Autodesk Inventor part; units mm, degrees
ref_plane "YZ Plane" through (0, 0, 0) normal (1, 0, 0) x (0, 1, 0)
ref_plane "XZ Plane" through (0, 0, 0) normal (0, 1, 0) x (-1, 0, 0)
ref_plane "XY Plane" through (0, 0, 0) normal (0, 0, 1) x (1, 0, 0)
sketch "Esboço1" plane through (0, 0, 0) normal (0, 0, 1) x (1, 0, 0)
  line L0 (0, 0) -> (100, 0)
  line L1 (100, 0) -> (100, -100)
  line L2 (100, -100) -> (0, -100)
  line L3 (0, -100) -> (0, 0)
  dimension "d0" = 100
  dimension "d1" = 100
extrude "Extrusão1" add sketch "Esboço1" along normal blind 3
sketch "Esboço2" plane through (0, 0, 3) normal (0, 0, 1) x (1, 0, 0)
  line L0 (0, 0) -> (0, -100)
  line L1 (0, 0) -> (9.75, 0)
  line L2 (100, 0) -> (0, 0)
  line L3 (9.75, 0) -> (9.75, -10)
  line L4 (9.75, 0) -> (21.25, 0)
  line L5 (21.25, 0) -> (32.75, 0)
  line L6 (32.75, 0) -> (44.25, 0)
  line L7 (44.25, 0) -> (55.75, 0)
  line L8 (55.75, 0) -> (67.25, 0)
  line L9 (67.25, 0) -> (78.75, 0)
  line L10 (78.75, 0) -> (90.25, 0)
  line L11 (90.25, 0) -> (100, 0)
  line L12 (21.25, 0) -> (21.25, -10)
  line L13 (9.75, -10) -> (9.75, -37.6)
  line L14 (9.75, -37.6) -> (21.25, -37.6)
  line L15 (21.25, -37.6) -> (32.75, -37.6)
  line L16 (32.75, -37.6) -> (44.25, -37.6)
  line L17 (44.25, -37.6) -> (55.75, -37.6)
  line L18 (55.75, -37.6) -> (67.25, -37.6)
  line L19 (67.25, -37.6) -> (78.75, -37.6)
  line L20 (78.75, -37.6) -> (90.25, -37.6)
  line L21 (90.25, -37.6) -> (90.25, -10)
  line L22 (90.25, -10) -> (78.75, -10)
  line L23 (78.75, -10) -> (67.25, -10)
  line L24 (67.25, -10) -> (55.75, -10)
  line L25 (55.75, -10) -> (44.25, -10)
  line L26 (44.25, -10) -> (32.75, -10)
  line L27 (32.75, -10) -> (21.25, -10)
  circle A0 centre (9.75, -10) radius 1.5
  circle A1 centre (9.75, -37.6) radius 1.5
  circle A2 centre (32.75, -10) radius 1.5
  circle A3 centre (55.75, -10) radius 1.5
  circle A4 centre (78.75, -10) radius 1.5
  circle A5 centre (78.75, -37.6) radius 1.5
  circle A6 centre (55.75, -37.6) radius 1.5
  circle A7 centre (32.75, -37.6) radius 1.5
  line L28 (21.25, -10) -> (21.25, -20)
  circle A8 centre (21.25, -20) radius 1.5
  line L29 (21.25, -20) -> (21.25, -47.6)
  line L30 (21.25, -47.6) -> (44.25, -47.6)
  line L31 (44.25, -47.6) -> (67.25, -47.6)
  line L32 (67.25, -47.6) -> (90.25, -47.6)
  line L33 (90.25, -47.6) -> (90.25, -20)
  line L34 (90.25, -20) -> (67.25, -20)
  line L35 (67.25, -20) -> (44.25, -20)
  circle A9 centre (21.25, -47.6) radius 1.5
  circle A10 centre (44.25, -47.6) radius 1.5
  circle A11 centre (67.25, -47.6) radius 1.5
  circle A12 centre (90.25, -47.6) radius 1.5
  circle A13 centre (90.25, -20) radius 1.5
  circle A14 centre (67.25, -20) radius 1.5
  circle A15 centre (44.25, -20) radius 1.5
  dimension "d4" = 9.75
  dimension "d5" = 10
  dimension "d7" = 11.5
  dimension "d8" = 11.5
  dimension "d9" = 11.5
  dimension "d10" = 11.5
  dimension "d11" = 11.5
  dimension "d12" = 11.5
  dimension "d13" = 11.5
  dimension "d14" = 27.6
  dimension "d16" = 3
  dimension "d17" = 3
  dimension "d19" = 3
  dimension "d21" = 3
  dimension "d23" = 3
  dimension "d26" = 3
  dimension "d28" = 3
  dimension "d30" = 3
  dimension "d101" = 10
  dimension "d102" = 3
  dimension "d103" = 27.6
  dimension "d104" = 23
  dimension "d105" = 23
  dimension "d106" = 23
  dimension "d107" = 27.6
  dimension "d108" = 23
  dimension "d109" = 23
  dimension "d110" = 3
  dimension "d111" = 3
  dimension "d112" = 3
  dimension "d113" = 3
  dimension "d114" = 3
  dimension "d115" = 3
  dimension "d116" = 3
extrude "Extrusão6" add sketch "Esboço2" along normal blind 15 contours A15 | A14 L35 L34 | L34 L35 A14 | A0 L13 L3 | L3 L13 A0 | A2 L26 L27 | L27 L26 A2 | A8 L29 L28 | L28 L29 A8 | A1 L14 L13 | L13 L14 A1 | A3 L24 L25 | L25 L24 A3 | A7 L16 L15 | L15 L16 A7 | A9 L30 L29 | L29 L30 A9 | A10 L31 L30 | L30 L31 A10 | A4 L22 L23 | L23 L22 A4 | A6 L18 L17 | L17 L18 A6 | A11 L32 L31 | L31 L32 A11 | A13 L21 | L21 L34 A13 | A5 L20 L19 | L19 L20 A5 | A12 L33 L32 | L32 L33 A12 | L21 A13 L34
sketch "Esboço5" plane through (9.75, -10, 18) normal (0, 0, 1) x (1, 0, 0)
  circle A0 centre (0, 0) radius 1.5
  line L0 (0, 0) -> (23, 0)
  line L1 (23, 0) -> (46, 0)
  line L2 (46, 0) -> (69, 0)
  line L3 (0, 0) -> (0, -27.6)
  line L4 (0, -27.6) -> (23, -27.6)
  line L5 (23, -27.6) -> (46, -27.6)
  line L6 (46, -27.6) -> (69, -27.6)
  line L7 (0, 0) -> (11.5, 0)
  line L8 (11.5, 0) -> (11.5, -10)
  line L9 (11.5, -10) -> (34.5, -10)
  line L10 (34.5, -10) -> (57.5, -10)
  line L11 (57.5, -10) -> (80.5, -10)
  line L12 (80.5, -10) -> (80.5, -37.6)
  line L13 (80.5, -37.6) -> (57.5, -37.6)
  line L14 (57.5, -37.6) -> (34.5, -37.6)
  circle A1 centre (34.5, -37.6) radius 1.5
  line L15 (34.5, -37.6) -> (11.5, -37.6)
  circle A2 centre (0, 0) radius 0.95
  circle A3 centre (11.5, -10) radius 0.95
  circle A4 centre (23, 0) radius 1.5
  circle A5 centre (23, 0) radius 0.95
  circle A6 centre (34.5, -10) radius 0.95
  circle A7 centre (46, 0) radius 1.5
  circle A8 centre (46, 0) radius 0.95
  circle A9 centre (57.5, -10) radius 0.95
  circle A10 centre (69, 0) radius 1.5
  circle A11 centre (69, 0) radius 0.95
  circle A12 centre (80.5, -10) radius 0.95
  circle A13 centre (69, -27.6) radius 0.95
  circle A14 centre (80.5, -37.6) radius 0.95
  circle A15 centre (57.5, -37.6) radius 0.95
  circle A16 centre (46, -27.6) radius 0.95
  circle A17 centre (34.5, -37.6) radius 0.95
  circle A18 centre (23, -27.6) radius 0.95
  circle A19 centre (11.5, -37.6) radius 0.95
  circle A20 centre (0, -27.6) radius 0.95
  point P0 (-9.75, 10)
  dimension "d119" = 23
  dimension "d120" = 23
  dimension "d121" = 23
  dimension "d122" = 27.6
  dimension "d123" = 23
  dimension "d124" = 23
  dimension "d125" = 23
  dimension "d126" = 11.5
  dimension "d127" = 10
  dimension "d128" = 23
  dimension "d129" = 23
  dimension "d130" = 23
  dimension "d131" = 27.6
  dimension "d132" = 23
  dimension "d133" = 23
  dimension "d134" = 23
extrude "Extrusão7" add sketch "Esboço5" along normal blind 10 contours A13 | A16 L6 L5 | L5 L6 A16 | A18 L5 L4 | L4 L5 A18 | A20 L4 L3 | L3 L4 A20 | A11 | A19 | A15 L14 L13 | L13 L14 A15 | A14 L13 L12 | L12 L13 A14 | A12 L12 L11 | L11 L12 A12 | A9 L11 L10 | L10 L11 A9 | A6 L10 L9 | L9 L10 A6 | A3 L9 L8 | L8 L9 A3 | A2 L3 L0 | L0 L3 A2 | A5 L1 L0 | L0 L1 A5 | A8 L2 L1 | L1 L2 A8 | A17 L15 L14 | L14 L15 A17
properties part number "Palma"
Geometry check sheet. Reference: the model listing, model coordinates, mm. A direction names the side the tool comes from. Give positions to 0.01 mm unless a question says otherwise; leave off trailing zeros. Order: outer loops, then holes, each group sorted by start corner. A loop starts at its lowest first (then second) coordinate and runs counter-clockwise, first axis right, second up.
1. Draft check along X on faces 1 (the face through (49, -49, 0)), 2 (the face through (0, -51, 1)), 3 (the face through (100, -49, 1)), 4 (the face through (57, -38, 18)). Enter one of: pulls with the +X half, pulls with the -X half, needs draft (parallel to the pull), parting line crosses it, or undercut.
Completed:
face 1: needs draft
face 2: pulls with the -X half
face 3: pulls with the +X half
face 4: undercut
2. Depth check by flat-ended pin: pin 1 (10 mm diameter, centred on x = 88.5, y = -62, fed in from +Z); pin 2 (10 mm diameter, centred on y = -17.5, z = 9.5, fed in from -X); pin 3 (6 mm diameter, centred on x = 20.5, z = 18.5, fed in from -Y). Enter the tip coordinate at first touch or a pass-through.
Completed:
pin 1: stops at z = 3
pin 2: stops at x = 19.75
pin 3: stops at y = -49.1
3. Sectioned sample at D-D (y = -44.5). Record the boundary of the cut face in (x, z), then the cut area to 3 significant figures.
Completed:
outline: (0, 0) - (100, 0) - (100, 3) - (0, 3) - close
area: 300 mm2
4. Sectioned sample at A-A (z = 10.25). State how many separate pieces and enclosed holes the cut face has, then the cut area to 3 significant figures.
Completed:
separate pieces: 16
enclosed holes: 0
area: 113 mm2
5. Scan lines: line 1 (Z direction, x = 86.5, y = -88.5); line 2 (Y direction, x = 91, z = 16); line 3 (Y direction, x = 68, z = 19.5). Record each from-to range of solid material in increasing order.
Completed:
line 1: z = 0 to 3
line 2: y = -48.9 to -46.3, -21.3 to -18.7
line 3: y = -48.18 to -47.02, -20.58 to -19.42
6. Access from +Z, -Z, +X, -X, +Y, -Y to the whole of each face (thin tool, end or side, straight path). Record for faces 5 (the face through (49, 0, 1)), 6 (the face through (34, -38, 18)).
Completed:
face 5: +Z, -Z, +X, -X, +Y
face 6: +Z
7. Sectioned sample at C-C (x = 39). Record the boundary of the cut face in (y, z), then the cut area to 3 significant figures.
Completed:
outline: (-100, 0) - (0, 0) - (0, 3) - (-100, 3) - close
area: 300 mm2
